```python
from build123d import *

# Parameters (mm, degrees)
F0_R        = 9.4742
F1_DEPTH    = 82.55
F2_R        = 9.4742
F3_DEPTH    = 2.286
F4_W        = 12.7000000767
F4_H        = 82.55
F4_W_2      = 12.7
F5_DEPTH    = 2.286
F6_T1_DEPTH = 82.55
F7_R        = 0.7874
F8_DEPTH    = 13.208


# Not quite as in the source:
# - a fillet or chamfer that OpenCascade refuses, or shapes differently, is made with other operations: its cross-section is extruded or revolved along the edge and cut away or added
# - a pattern or mirror of a feature is missing from the dataset's text; its kind, count and spacing are read off the source's solid


with BuildPart() as f1:
    # F0 (on Top) → F1 (new body)
    with BuildSketch(Plane.XY):
        with BuildLine():
            ThreePointArc((-11.049, -6.3499999233), (-9.4295157118, -6.785458523), (-7.9847846533, -7.6369899201))
            ThreePointArc((-7.9847846533, -7.6369899201), (-7.5622828297, -8.001877119), (-7.1741300574, -8.4031100742))
            ThreePointArc((-7.1741300574, -8.4031100742), (11.0467672464, 0.2221134929), (-7.5061119691, 8.1079395723))
            ThreePointArc((-7.5061119691, 8.1079395723), (-7.6290075774, 7.9871909027), (-7.755263928, 7.8699607628))
            ThreePointArc((-7.755263928, 7.8699607628), (-9.2865444962, 6.859503776), (-11.049, 6.35))
            ThreePointArc((-11.049, 6.35), (-11.84275, 6.2981423564), (-12.6365, 6.35))
            Line((-12.6365, 6.35), (-14.224, 6.35))
            Line((-14.224, 6.35), (-14.224, -6.3499999233))
            Line((-14.224, -6.3499999233), (-12.6365, -6.3499999233))
            ThreePointArc((-12.6365, -6.3499999233), (-11.84275, -6.2992439038), (-11.049, -6.3499999233))
        make_face()
        Circle(F0_R, mode=Mode.SUBTRACT)
    extrude(amount=F1_DEPTH)

    # F2 (on face) → F3 (join)
    with BuildSketch(Plane(origin=(0, 0, 0), x_dir=(1, 0, 0), z_dir=(0, 0, -1))):
        Circle(F2_R)
    extrude(amount=-F3_DEPTH)

    # F4 (on face) → F5 (join)
    with BuildSketch(Plane(origin=(-14.224, 0, 0), x_dir=(0, -1, 0), z_dir=(-1, 0, 0))):
        Polygon((6.3499999233, 82.55), (0, 82.55), (-6.35, 82.55), (-6.35, 0), (6.3499999233, 0), align=None)
        with Locations((12.6999999616, 41.275)):
            Rectangle(F4_W, F4_H)
        with Locations((-12.7, 41.275)):
            Rectangle(F4_W_2, F4_H)
    extrude(amount=F5_DEPTH)

    # F6: fillet of radius 3.048 on 2 edges, made by hand

    # F6_s2 → F6_t1 (join)
    with BuildSketch(Plane.XY):
        with BuildLine():
            ThreePointArc((-14.224, -9.0253024762), (-13.7972504649, -7.4698764896), (-12.6365, -6.3499999233))
            Line((-12.6365, -6.3499999233), (-14.224, -6.3499999233))
            Line((-14.224, -6.3499999233), (-14.224, -9.0253024762))
        make_face()
        with BuildLine():
            ThreePointArc((-14.224, 9.025302553), (-13.7972504649, 7.4698765663), (-12.6365, 6.35))
            Line((-12.6365, 6.35), (-14.224, 6.35))
            Line((-14.224, 6.35), (-14.224, 9.025302553))
        make_face()
    extrude(amount=F6_T1_DEPTH)

    # F7 (on face) → F8 (cut)
    with BuildSketch(Plane.YZ.offset(-14.224)):
        with Locations((-14.0376512381, 70.7353055477)):
            Circle(F7_R)
        with Locations((-14.0376512381, 12.7)):
            Circle(F7_R)
    f8 = extrude(amount=-F8_DEPTH, mode=Mode.SUBTRACT)

    # F8_copies: F8 across plane
    add(f8.mirror(Plane.ZX), mode=Mode.SUBTRACT)


solid = f1.part
```
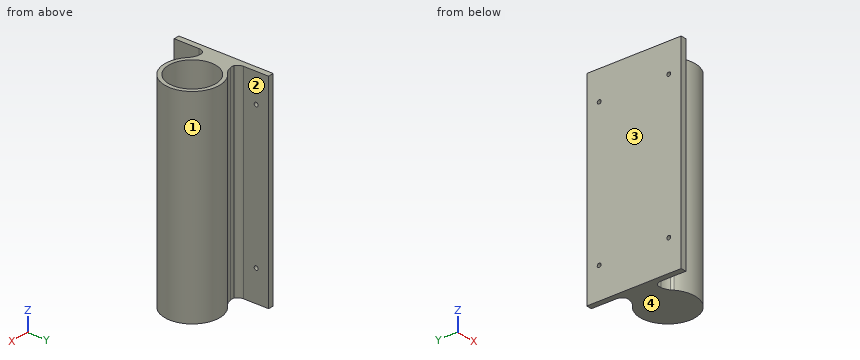
Geometry check sheet. Reference: the model listing, model coordinates, mm. Face numbers are marked on the shaded views. Coordinates: 2 decimals unless noted, no trailing zeros. Order: outer loops, then holes, each group sorted by start corner. A loop starts at its lowest first (then second) coordinate and runs counter-clockwise, first axis right, second up. Notation, with made-up numbers: M -31,7 L -3,7 A15 ccw -3,14 Z; hole C 30.5,27 d11. An arc over 180 degrees is marked long. Answer as a JSON object with one key per item and string values.
Q1. Cross-section at C-C on z = 61. Record the cut outline in (x, y).
Results are:
{"outline": "M -16.51,-19.05 L -14.22,-19.05 L -14.22,-9.03 A3.05 cw -12.64,-6.35 A6.23 cw -7.17,-8.4 A11.05 ccw long -7.51,8.11 A6.1 cw -12.64,6.35 A3.05 cw -14.22,9.03 L -14.22,19.05 L -16.51,19.05 Z; hole C 0,0 d18.95"}
Q2. Cross-section at A-A on z = 12.7. Record the cut outline in (x, y), and give its area (3 significant figures).
Results are:
{"outline": "M -16.51,-19.05 L -14.22,-19.05 L -14.22,-14.83 L -16.51,-14.83 Z; M -16.51,-13.25 L -14.22,-13.25 L -14.22,-9.03 A3.05 cw -12.64,-6.35 A6.23 cw -7.17,-8.4 A11.05 ccw long -7.51,8.11 A6.1 cw -12.64,6.35 A3.05 cw -14.22,9.03 L -14.22,13.25 L -16.51,13.25 Z; M -16.51,14.83 L -14.22,14.83 L -14.22,19.05 L -16.51,19.05 Z; hole C 0,0 d18.95", "area": "234 mm²"}
Q3. Cross-section at D-D on y = 0. Record the cut outline in (x, z), and give its area (3 significant figures).
Results are:
{"outline": "M -16.51,0 L 11.05,0 L 11.05,82.55 L 9.47,82.55 L 9.47,2.29 L -9.47,2.29 L -9.47,82.55 L -16.51,82.55 Z", "area": "754 mm²"}
Q4. Scan lines: line 1 (Y direction, x = -0.25, z = 23); line 2 (X direction, y = -0.5, z = 7); line 3 (X direction, y = -7, z = 33). Record each from-to range of solid material in increasing order.
Results are:
{"line 1": "y = -11.05 to -9.47, 9.47 to 11.05", "line 2": "x = -16.51 to -9.46, 9.46 to 11.04", "line 3": "x = -16.51 to -13.45, -8.97 to -6.38, 6.38 to 8.55"}
Q5. Cross-section at B-B on x = 0. Record the cut outline in (y, z).
Results are:
{"outline": "M -11.05,0 L 11.05,0 L 11.05,82.55 L 9.47,82.55 L 9.47,2.29 L -9.47,2.29 L -9.47,82.55 L -11.05,82.55 Z"}
Q6. Depth check by flat-ended pin: pin 1 Ø1.5 at (x, z) = (-9.5, 63.5) entering from +Y; pin 2 Ø3 at (y, z) = (14, 27) entering from +X; pin 3 Ø1.5 at (y, z) = (-1.5, 26) entering from +X. Enter the tip coordinate at first touch or a pass-through.
Results are:
{"pin 1": "stops at y = 7.14", "pin 2": "stops at x = -14.22", "pin 3": "stops at x = 11.02"}
Q7. Release check for a two-part mould opening along X. For the marked faces 1, 2, 3 and 4 record: released by +X, released by -X, zero draft, split by the parting line, or undercut.
Results are:
{"face 1": "undercut", "face 2": "undercut", "face 3": "released by -X", "face 4": "zero draft"}
